For this review, take the finished solid that the model builds, in its own axes (mm). A direction names the side the tool comes from. Give positions to 0.01 mm unless a question says otherwise; leave off trailing zeros. Write each loop counter-clockwise with the first axis right and the second up, starting at its lowest first coordinate (ties: lowest second). Pieces come first, ordered by that corner, then holes.
Q1. Mouldability with a two-part tool opening along X and no side actions: class faces 4 (the flat face through (0, 3, 0)), 5 (the cylindrical face through (2.87, 1.52, -7.87)), 6 (the flat face through (0, 1, 12.63)) as released by +X, released by -X, zero draft, split by the parting line, or undercut.
Q2. We need section C-C (y = 5.5). Write out the cut boundary in (x, z) (3 decimals).
Q3. Machinability: for faces 1 (the cylindrical face through (-7.9, 1.52, 2.85)), 2 (the cylindrical face through (-8.416, 1.479, -0.363)), 3 (the flat face through (-3, 6.2, 7)), which of the approach directions +Z, -Z, +X, -X, +Y, -Y give a long, thin tool a straight path to every point of the face, cutting with its end or side? Answer none if there is none.
Q4. Insertion check: P1, Ø9.5, axis at x = -1, z = -5.5, coming from the -Y side; P2, Ø3, axis at x = 0, z = -9.57, coming from the +Y side; P3, Ø1, axis at x = -4.5, y = 11.5, coming from the +Z side; P4, Ø1, axis at x = -13, z = 8, coming from the +Y side. Each pin has a flat end and moves straight along its axis. Give the tip position at first contact, or say it passes through.
Q5. We need section A-A (x = 0). Give the number of separate pieces and of enclosed holes in the cut face, then the cut area to 3 significant figures.
Q6. For line 1 (Z direction, x = 9.57, y = 1.65) (3 decimals); line 2 (Y direction, x = 6, z = -1), list the stretches that pass through material, from the lowest coordinate up.
```python
from build123d import *

# Parameters (mm, degrees)
SKETCH1_R                = 8.03
SKETCH1_R_2              = 6.26
BOSS_EXTRUDE1_DEPTH      = 3
SKETCH1_4_R              = 1.21
BOSS_EXTRUDE3_DEPTH      = 3
FILLET1_R                = 2
CIRPATTERN1_COUNT        = 4
FILLET1_OF_CIRPATTERN1_R = 2
BOSS_EXTRUDE4_START      = 3
SKETCH1_5_R              = 7.145
SKETCH1_5_R_2            = 6.26
SKETCH1_5_R_3            = 2.475
BOSS_EXTRUDE4_DEPTH      = 3.2
BOSS_EXTRUDE5_START      = 6.2
SKETCH1_6_R              = 16.97
BOSS_EXTRUDE5_DEPTH      = 14.85
BOSS_EXTRUDE6_START      = 21.05
SKETCH1_7_R              = 2.475
BOSS_EXTRUDE6_DEPTH      = 13.86
FILLET3_SIZE             = 3
FILLET3_SIZE_2           = 1


with BuildPart() as part:
    # Sketch1 → Boss-Extrude1 (new body)
    with BuildSketch(Plane(origin=(0, 0, 0), x_dir=(1, 0, 0), z_dir=(0, 1, 0))):
        with Locations(Location((0, 0, 0), (0, 0, 270))):
            Circle(SKETCH1_R)
        with Locations(Location((0, 0, 0), (0, 0, 270))):
            Circle(SKETCH1_R_2, mode=Mode.SUBTRACT)
    extrude(amount=BOSS_EXTRUDE1_DEPTH)

    # Sketch1<4> → Boss-Extrude3 (add)
    with BuildSketch(Plane(origin=(0, 0, 0), x_dir=(1, 0, 0), z_dir=(0, 1, 0))):
        with BuildLine():
            Line((-2.565, 12.63), (-2.565, 7.609315015))
            ThreePointArc((-2.565, 7.609315015), (0, 8.03), (2.565, 7.609315015))
            Line((2.565, 7.609315015), (2.565, 12.63))
            Line((2.565, 12.63), (-2.565, 12.63))
        make_face()
        with Locations(Location((0, 9.57, 0), (0, 0, 270))):
            Circle(SKETCH1_4_R, mode=Mode.SUBTRACT)
    boss_extrude3 = extrude(amount=BOSS_EXTRUDE3_DEPTH)

    # Fillet1
    fillet1_edges = [part.edges().sort_by_distance(p)[0] for p in [
        (-2.565, 1.5, -7.609315015),
        (2.565, 1.5, -7.609315015),
        (2.565, 1.5, -12.63),
        (-2.565, 1.5, -12.63),
    ]]
    fillet(fillet1_edges, radius=FILLET1_R)

    # CirPattern1: Boss-Extrude3 ×4 about axis
    cirpattern1_axis = Axis((0, 0, 0), (0, 1, 0))
    for i in range(1, CIRPATTERN1_COUNT):
        add(boss_extrude3.rotate(cirpattern1_axis, i * 360 / CIRPATTERN1_COUNT))

    # Fillet1 of CirPattern1
    fillet1_of_cirpattern1_edges = [part.edges().sort_by_distance(p)[0] for p in [
        (-7.609315015, 1.5, 2.565),
        (-7.609315015, 1.5, -2.565),
        (-12.63, 1.5, -2.565),
        (-12.63, 1.5, 2.565),
        (2.565, 1.5, 7.609315015),
        (-2.565, 1.5, 7.609315015),
        (-2.565, 1.5, 12.63),
        (2.565, 1.5, 12.63),
        (7.609315015, 1.5, -2.565),
        (7.609315015, 1.5, 2.565),
        (12.63, 1.5, 2.565),
        (12.63, 1.5, -2.565),
    ]]
    fillet(fillet1_of_cirpattern1_edges, radius=FILLET1_OF_CIRPATTERN1_R)

    # Sketch1<5> → Boss-Extrude4 (add)
    # profile 1 of 3: a face of its own
    with BuildSketch(Plane(origin=(0, 0, 0), x_dir=(1, 0, 0), z_dir=(0, 1, 0)).offset(BOSS_EXTRUDE4_START)):
        with Locations(Location((0, 0, 0), (0, 0, 270))):
            Circle(SKETCH1_5_R)
        with Locations(Location((0, 0, 0), (0, 0, 270))):
            Circle(SKETCH1_5_R_2, mode=Mode.SUBTRACT)
    # profile 2 of 3: a face of its own
    with BuildSketch(Plane(origin=(0, 0, 0), x_dir=(1, 0, 0), z_dir=(0, 1, 0)).offset(BOSS_EXTRUDE4_START)):
        with Locations(Location((0, 0, 0), (0, 0, 270))):
            Circle(SKETCH1_5_R_2)
        Circle(SKETCH1_5_R_3, mode=Mode.SUBTRACT)
    # profile 3 of 3: a face of its own
    with BuildSketch(Plane(origin=(0, 0, 0), x_dir=(1, 0, 0), z_dir=(0, 1, 0)).offset(BOSS_EXTRUDE4_START)):
        Circle(SKETCH1_5_R_3)
    extrude(amount=BOSS_EXTRUDE4_DEPTH)

    # Sketch1<6> → Boss-Extrude5 (add)
    with BuildSketch(Plane(origin=(0, 0, 0), x_dir=(1, 0, 0), z_dir=(0, 1, 0)).offset(BOSS_EXTRUDE5_START)):
        with Locations(Location((0, 0, 0), (0, 0, 270))):
            Circle(SKETCH1_6_R)
    extrude(amount=BOSS_EXTRUDE5_DEPTH)

    # Sketch1<7> → Boss-Extrude6 (add)
    with BuildSketch(Plane(origin=(0, 0, 0), x_dir=(1, 0, 0), z_dir=(0, 1, 0)).offset(BOSS_EXTRUDE6_START)):
        with Locations(Location((0, 0, 0), (0, 0, 90))):
            Circle(SKETCH1_7_R)
    extrude(amount=BOSS_EXTRUDE6_DEPTH)

    # Sketch2 → Cut-Revolve2 (revolve, cut)
    with BuildSketch(Plane.XY, mode=Mode.PRIVATE) as cut_revolve2_sk:
        with BuildLine():
            add(Edge.make_bspline(
                [(10.47, 21.05), (15.814758039, 21.05), (16.969999933, 15.844909447), (16.97, 11.464372124)],
                knots=[0, 0, 0, 0, 0.661851635, 0.661851635, 0.661851635, 0.661851635], degree=3))
            Line((16.97, 11.464372124), (16.97, 21.05))
            Line((16.97, 21.05), (10.47, 21.05))
        make_face()
    revolve(cut_revolve2_sk.sketch.rotate(Axis((0, 21.05, 0), (0, -1, 0)), 90), axis=Axis((0, 21.05, 0), (0, -1, 0)), mode=Mode.SUBTRACT)

    # Fillet3
    # an asymmetric fillet: 3, 1 mm, written as the material it takes off along each edge
    with BuildSketch(Plane(origin=(0, 6.2, 0), x_dir=(0, 0, 1), z_dir=(-1, 0, 0))) as fillet3_piece_1:
        with BuildLine():
            Bezier((16.97, FILLET3_SIZE), (16.97, 0), (16.97 - FILLET3_SIZE_2, 0), weights=[1, 0.707106781, 1])
            Line((16.97 - FILLET3_SIZE_2, 0), (16.97, 0))
            Line((16.97, 0), (16.97, FILLET3_SIZE))
        make_face()
    revolve(axis=Axis((0, 6.2, 0), (0, 1, 0)), mode=Mode.SUBTRACT)


solid = part.part
```
Computed:
1. face 4: undercut
1. face 5: released by +X
1. face 6: zero draft
2. outline: circle Ø14.29 at (0, 0)
3. face 1: +Z, -X, -Y
3. face 2: -Y
3. face 3: none
4. P1: stops at y = 0
4. P2: stops at y = 21.05
4. P3: stops at z = 16.49
4. P4: stops at y = 19.3
5. separate pieces: 3
5. enclosed holes: 0
5. area: 619 mm2
6. line 1: z = -2.565 to -1.21, 1.21 to 2.565
6. line 2: y = 3 to 21.05
